from build123d import *

# Parameters (mm, degrees)
F0_R     = 15.24
F1_DEPTH = 31.75
F2_SIZE  = 3.81
F3_R     = 5.08


# Not quite as in the source:
# - a feature names something its author has since deleted; it is built from what else it names


with BuildPart() as f1:
    # F0 (on Top) → F1 (new body)
    with BuildSketch(Plane.XY):
        with BuildLine():
            ThreePointArc((19.05, -21.59), (34.3164354058, -15.2664354058), (40.64, 0))
            ThreePointArc((40.64, 0), (34.316284436, 15.2665863742), (19.0495729948, 21.5899999958))
            ThreePointArc((19.0495729948, 21.5899999958), (3.7834136258, 15.266284436), (-2.54, 0))
            ThreePointArc((-2.54, 0), (3.7835645942, -15.2664354058), (19.05, -21.59))
        make_face()
        with Locations((19.05, 0)):
            Circle(F0_R, mode=Mode.SUBTRACT)
        with BuildLine():
            Line((-24.13, -21.59), (19.05, -21.59))
            ThreePointArc((19.05, -21.59), (3.7835645942, -15.2664354058), (-2.54, 0))
            ThreePointArc((-2.54, 0), (-8.8635645942, -15.2664354058), (-24.13, -21.59))
        make_face()
        with BuildLine():
            ThreePointArc((-24.13, -21.59), (-8.8635645942, -15.2664354058), (-2.54, 0))
            ThreePointArc((-2.54, 0), (-8.7959724103, 15.1985426235), (-23.9383972097, 21.5891497834))
            ThreePointArc((-23.9383972097, 21.5891497834), (-45.7197874448, 0.0958023383), (-24.13, -21.59))
        make_face()
        with Locations((-24.13, 0)):
            Circle(F0_R, mode=Mode.SUBTRACT)
        with BuildLine():
            ThreePointArc((-2.54, 0), (3.7834136258, 15.266284436), (19.0495729948, 21.5899999958))
            Line((19.0495729948, 21.5899999958), (-23.9383972097, 21.5891497834))
            ThreePointArc((-23.9383972097, 21.5891497834), (-8.7959724103, 15.1985426235), (-2.54, 0))
        make_face()
    extrude(amount=F1_DEPTH)

    # F2
    f2_edges = [f1.edges().sort_by_distance(p)[0] for p in [
        (-39.37, 0, 0),
        (3.81, 0, 0),
        (3.81, 0, 31.75),
        (-39.37, 0, 31.75),
    ]]
    chamfer(f2_edges, length=F2_SIZE)

    # F3
    f3_edges = [f1.edges().sort_by_distance(p)[0] for p in [
        (-39.37, 0, 3.81),
        (-39.37, 0, 27.94),
        (3.81, 0, 27.94),
        (3.81, 0, 3.81),
    ]]
    fillet(f3_edges, radius=F3_R)


solid = f1.part
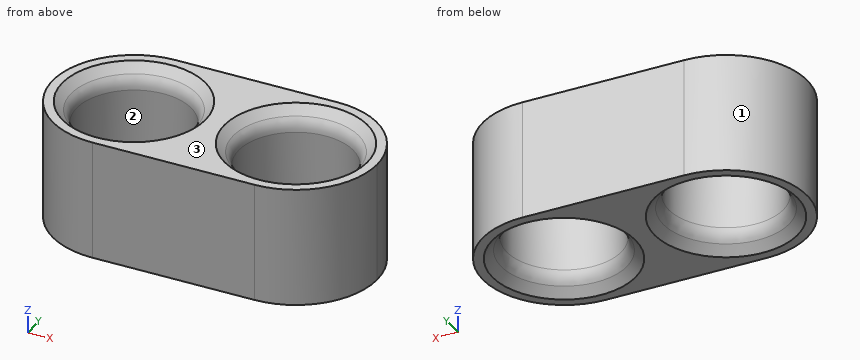
Source: CAD feature listing. Evaluate the final solid. Frame: model axes, mm. Face numbers are marked on the shaded views. Give positions to 0.01 mm unless a question says otherwise; leave off trailing zeros. Write each loop counter-clockwise with the first axis right and the second up, starting at its lowest first coordinate (ties: lowest second). Pieces come first, ordered by that corner, then holes. Notation, with made-up numbers: (-35, -37) - (17, -37) arc R19 ccw to (17, -29) - close; hole circle Ø4 at (62, 71). An arc over 180 degrees is marked (long way). Write item = value, one per line. Start each with the question number.
Q1. Cut plane A-A, the plane z = 20.5. Return loops of the section in (x, y).
Q2. Pin query (flat end, axial travel): pin 1 Ø8 at (y, z) = (12.5, 26) entering from +X; pin 2 Ø4 at (x, z) = (28, 16) entering from -Y. Return the tip coordinate at first contact, or that it passes through.
Q3. Draft query along Y for the marked faces 1, 2 and 3. Return one class per face: +Y half, -Y half, draft (parallel to the pull), parting line (faces both ways), or undercut.
Q4. Cut plane B-B, the plane y = 10. Give the number of separate pieces and of enclosed holes in the cut face, then the cut area to 3 significant figures.
Q5. Material intervals for probe 1 along Y at (x, z) = (-24.13, 14.75); probe 2 along X at (y, z) = (-7.5, 4); probe 3 along X at (y, z) = (-0.5, 3), sorted ascending.
Computed values:
q1.outline = (-24.13, -21.59) - (19.05, -21.59) arc R21.59 ccw to (19.05, 21.59) - (-23.94, 21.59) arc R21.59 ccw (long way) to start; hole circle Ø30.48 at (-24.13, 0); hole circle Ø30.48 at (19.05, 0)
q2.pin_1 = 38.9
q2.pin_2 = -20.44
q3.face_1 = parting line
q3.face_2 = undercut
q3.face_3 = draft
q4.separate_pieces = 3
q4.enclosed_holes = 0
q4.area = 1,050 mm²
q5.probe_1 = -21.59 to -15.24, 15.24 to 21.59
q5.probe_2 = -44.38 to -37.83, -10.43 to 5.35, 32.75 to 39.3
q5.probe_3 = -45.71 to -40.28, -7.98 to 2.9, 35.2 to 40.63
